Geometry: see drawing. Coordinates: mm, zero at the bounding-box minimum. A direction names the side the tool comes from. Give positions to 0.01 mm unless a question says otherwise; leave off trailing zeros. Order: outer loops, then holes, each group sorted by start corner. A loop starts at its lowest first (then second) coordinate and runs counter-clockwise, first axis right, second up. Notation, with made-up numbers: M -3.75,15 L 27.25,15 A24 ccw 27.25,35 Z; hole C -17.75,37.5 d2. An arc over 180 degrees is marked long. Write item = value, one per line. Start each with the question number.
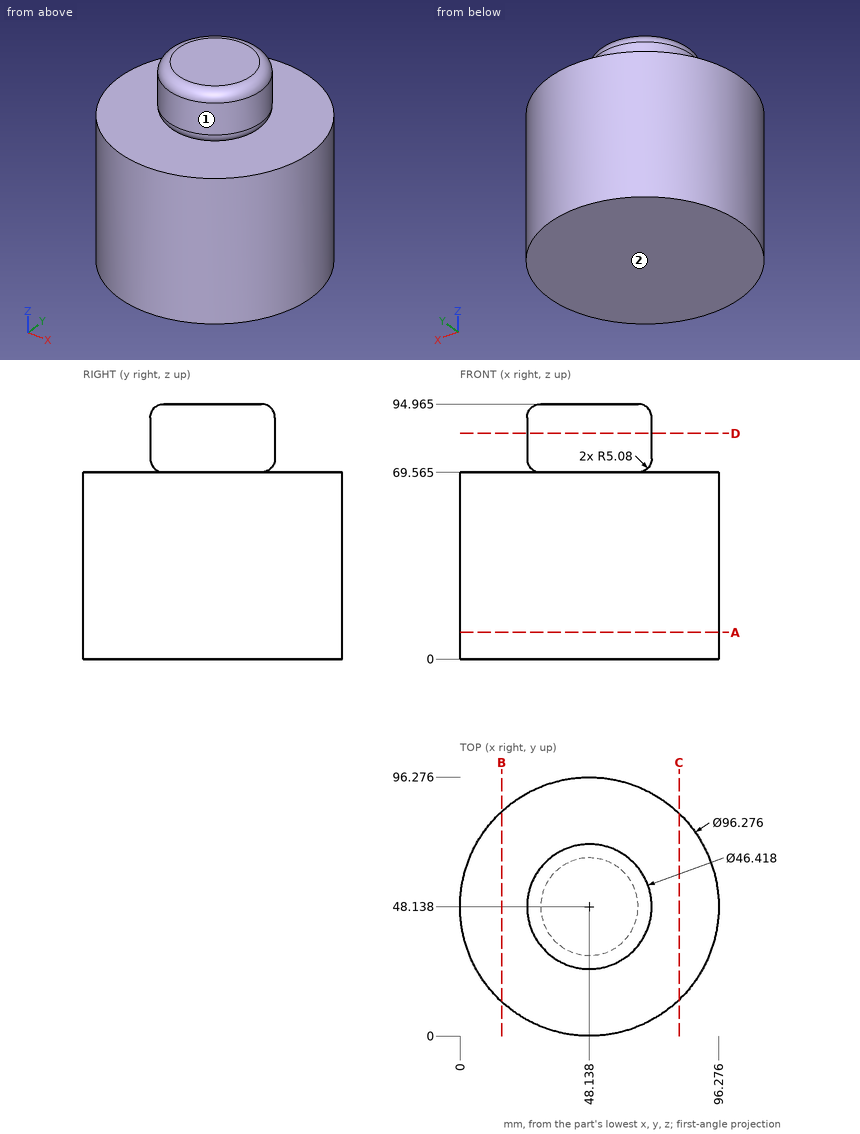
1) Ray query, L1, parallel to Z at x = 11, y = 25 (1 decimal); L2, parallel to X at y = 21, z = 37; L3, parallel to X at y = 89.5, z = 68.5 (1 decimal). Return the intervals inside material, ascending.
2) Cut plane D-D (z = 84). Return loops of the section in (x, y).
3) Cut plane C-C (x = 81.5). Return loops of the section in (y, z) (1 decimal), plus the area to 3 significant figures.
4) Cut plane B-B (x = 15.5). Return loops of the section in (y, z) (1 decimal), plus the area to 3 significant figures.
5) Cut plane A-A (z = 10). Return loops of the section in (x, y), plus the area to 3 significant figures.
6) Pin query (flat end, axial travel): pin 1 Ø2 at (x, y) = (55, 68.5) entering from +Z (1 decimal); pin 2 Ø8 at (x, y) = (19.5, 44) entering from -Z; pin 3 Ø10 at (y, z) = (31, 45.5) entering from +X; pin 4 Ø12 at (x, y) = (62, 76.5) entering from +Z (1 decimal). Return the tip coordinate at first contact, or that it passes through.
7) Access query for the marked faces 1 and 2. Directions: +Z, -Z, +X, -X, +Y, -Y. A direction counts if a zero-diameter tool reaches every point of the face in a straight line with its end or side. Return the directions, or none.
Reply:
q1.L1 = 0 to 69.6
q1.L2 = 8.38 to 87.9
q1.L3 = 23.5 to 72.8
q2.outline = C 48.14,48.14 d46.42
q3.outline = M 13.4,0 L 82.8,0 L 82.8,69.6 L 13.4,69.6 Z
q3.area = 4,830 mm²
q4.outline = M 12.8,0 L 83.5,0 L 83.5,69.6 L 12.8,69.6 Z
q4.area = 4,920 mm²
q5.outline = C 48.14,48.14 d96.28
q5.area = 7,280 mm²
q6.pin_1 = 94.4
q6.pin_2 = 0
q6.pin_3 = 94.72
q6.pin_4 = 69.6
q7.face_1 = +Z
q7.face_2 = -Z, +X, -X, +Y, -Y
